from build123d import *

# Parameters (mm, degrees)
SKETCH1_R                = 150
BOSS_EXTRUDE1_DEPTH      = 75
CHAMFER1_SIZE            = 10
BOSS_EXTRUDE2_START      = -65
BOSS_EXTRUDE2_DEPTH      = 10
CHAMFER2_SIZE            = 7
BOSS_EXTRUDE3_DEPTH      = 9
BOSS_EXTRUDE4_DEPTH      = 3.5
CIRPATTERN1_COUNT        = 4
CIRPATTERN1_COPY_1_DEPTH = 9
CIRPATTERN1_COPY_2_DEPTH = 9
CIRPATTERN1_COPY_3_DEPTH = 9
CIRPATTERN1_COPY_4_DEPTH = 3.5
CIRPATTERN1_COPY_5_DEPTH = 3.5
CIRPATTERN1_COPY_6_DEPTH = 3.5
CUT_EXTRUDE1_START       = -60
CUT_EXTRUDE1_DEPTH       = 60
SKETCH6_R                = 110
BOSS_EXTRUDE5_DEPTH      = 9
BOSS_EXTRUDE5_TAPER      = 45
SKETCH7_R                = 15
BOSS_EXTRUDE6_DEPTH      = 20


with BuildPart() as part:
    # Sketch1 → Boss-Extrude1 (new body)
    with BuildSketch(Plane(origin=(0, 0, 0), x_dir=(1, 0, 0), z_dir=(0, 1, 0))):
        with Locations(Location((0, 0, 0), (0, 0, 270))):
            Circle(SKETCH1_R)
    extrude(amount=BOSS_EXTRUDE1_DEPTH)

    # Chamfer1
    chamfer1_edges = [part.edges().sort_by_distance(p)[0] for p in [
        (0, 75, -150),
    ]]
    chamfer(chamfer1_edges, length=CHAMFER1_SIZE)

    # Sketch2 → Boss-Extrude2 (add)
    with BuildSketch(Plane(origin=(0, 75, 0), x_dir=(1, 0, 0), z_dir=(0, 1, 0)).offset(BOSS_EXTRUDE2_START)):
        with BuildLine():
            Line((-145.236875483, 37.5), (-195.236875483, 37.5))
            Line((-195.236875483, 37.5), (-195.236875483, -37.5))
            Line((-195.236875483, -37.5), (-145.236875483, -37.5))
            ThreePointArc((-145.236875483, -37.5), (-150, 0), (-145.236875483, 37.5))
        make_face()
    boss_extrude2 = extrude(amount=BOSS_EXTRUDE2_DEPTH)

    # Chamfer2
    chamfer2_edges = [part.edges().sort_by_distance(p)[0] for p in [
        (-195.236875483, 15, -37.5),
        (-195.236875483, 15, 37.5),
    ]]
    chamfer(chamfer2_edges, length=CHAMFER2_SIZE)

    # Sketch3 → Boss-Extrude3 (add)
    with BuildSketch(Plane.XY.offset(37.5)):
        Polygon((-145.236875483, 20), (-145.236875483, 65), (-170.556875483, 65), (-188.236875483, 20), align=None)
    boss_extrude3 = extrude(amount=-BOSS_EXTRUDE3_DEPTH)

    # Sketch4 → Boss-Extrude4 (add)
    with BuildSketch(Plane(origin=(0, 20, 0), x_dir=(1, 0, 0), z_dir=(0, 1, 0))):
        Polygon((-183.04072306, -12), (-188.236875483, -9), (-193.433027905, -12), (-193.433027905, -18), (-188.236875483, -21), (-183.04072306, -18), align=None)
    boss_extrude4 = extrude(amount=BOSS_EXTRUDE4_DEPTH)

    # Mirror1: Boss-Extrude3, Boss-Extrude4 across plane
    add(boss_extrude3.mirror(Plane.XY))
    add(boss_extrude4.mirror(Plane.XY))

    # CirPattern1: Boss-Extrude2, Boss-Extrude3, Boss-Extrude4 ×4 about axis
    cirpattern1_axis = Axis((0, 0, 0), (0, 1, 0))
    add([boss_extrude2.rotate(cirpattern1_axis, i * 360 / CIRPATTERN1_COUNT) for i in range(1, CIRPATTERN1_COUNT)])
    add([boss_extrude3.rotate(cirpattern1_axis, i * 360 / CIRPATTERN1_COUNT) for i in range(1, CIRPATTERN1_COUNT)])
    add([boss_extrude4.rotate(cirpattern1_axis, i * 360 / CIRPATTERN1_COUNT) for i in range(1, CIRPATTERN1_COUNT)])

    # CirPattern1 copy 1 sketch → CirPattern1 copy 1 (add)
    with BuildSketch(Plane(origin=(-37.5, 0, 0), x_dir=(0, 0, -1), z_dir=(-1, 0, 0))):
        Polygon((-145.236875483, -20), (-145.236875483, -65), (-170.556875483, -65), (-188.236875483, -20), align=None)
    extrude(amount=-CIRPATTERN1_COPY_1_DEPTH)

    # CirPattern1 copy 2 sketch → CirPattern1 copy 2 (add)
    with BuildSketch(Plane(origin=(0, 0, 37.5), x_dir=(-1, 0, 0), z_dir=(0, 0, 1))):
        Polygon((-145.236875483, -20), (-145.236875483, -65), (-170.556875483, -65), (-188.236875483, -20), align=None)
    extrude(amount=-CIRPATTERN1_COPY_2_DEPTH)

    # CirPattern1 copy 3 sketch → CirPattern1 copy 3 (add)
    with BuildSketch(Plane(origin=(37.5, 0, 0), x_dir=(0, 0, 1), z_dir=(1, 0, 0))):
        Polygon((-145.236875483, -20), (-145.236875483, -65), (-170.556875483, -65), (-188.236875483, -20), align=None)
    extrude(amount=-CIRPATTERN1_COPY_3_DEPTH)

    # CirPattern1 copy 4 sketch → CirPattern1 copy 4 (add)
    with BuildSketch(Plane(origin=(0, 20, 0), x_dir=(0, 0, -1), z_dir=(0, 1, 0))):
        Polygon((-183.04072306, 12), (-188.236875483, 9), (-193.433027905, 12), (-193.433027905, 18), (-188.236875483, 21), (-183.04072306, 18), align=None)
    extrude(amount=CIRPATTERN1_COPY_4_DEPTH)

    # CirPattern1 copy 5 sketch → CirPattern1 copy 5 (add)
    with BuildSketch(Plane(origin=(0, 20, 0), x_dir=(-1, 0, 0), z_dir=(0, 1, 0))):
        Polygon((-183.04072306, 12), (-188.236875483, 9), (-193.433027905, 12), (-193.433027905, 18), (-188.236875483, 21), (-183.04072306, 18), align=None)
    extrude(amount=CIRPATTERN1_COPY_5_DEPTH)

    # CirPattern1 copy 6 sketch → CirPattern1 copy 6 (add)
    with BuildSketch(Plane.ZX.offset(20)):
        Polygon((-183.04072306, 12), (-188.236875483, 9), (-193.433027905, 12), (-193.433027905, 18), (-188.236875483, 21), (-183.04072306, 18), align=None)
    extrude(amount=CIRPATTERN1_COPY_6_DEPTH)

    # Sketch5 → Cut-Extrude1 (cut)
    with BuildSketch(Plane(origin=(0, 75, 0), x_dir=(1, 0, 0), z_dir=(0, 1, 0)).offset(CUT_EXTRUDE1_START)):
        with BuildLine():
            Line((-112.583302492, -65), (-129.903810568, -75))
            ThreePointArc((-129.903810568, -75), (-106.066017178, -106.066017178), (-75, -129.903810568))
            Line((-75, -129.903810568), (-65, -112.583302492))
            ThreePointArc((-65, -112.583302492), (-91.923881554, -91.923881554), (-112.583302492, -65))
        make_face()
    extrude(amount=CUT_EXTRUDE1_DEPTH, mode=Mode.SUBTRACT)

    # Sketch6 → Boss-Extrude5 (add)
    with BuildSketch(Plane(origin=(0, 75, 0), x_dir=(1, 0, 0), z_dir=(0, 1, 0))):
        Circle(SKETCH6_R)
    extrude(amount=BOSS_EXTRUDE5_DEPTH, taper=BOSS_EXTRUDE5_TAPER)

    # Sketch7 → Boss-Extrude6 (add)
    with BuildSketch(Plane(origin=(0, 84, 0), x_dir=(1, 0, 0), z_dir=(0, 1, 0))):
        with Locations(Location((0, 0, 0), (0, 0, 270))):
            Circle(SKETCH7_R)
    extrude(amount=BOSS_EXTRUDE6_DEPTH)


solid = part.part
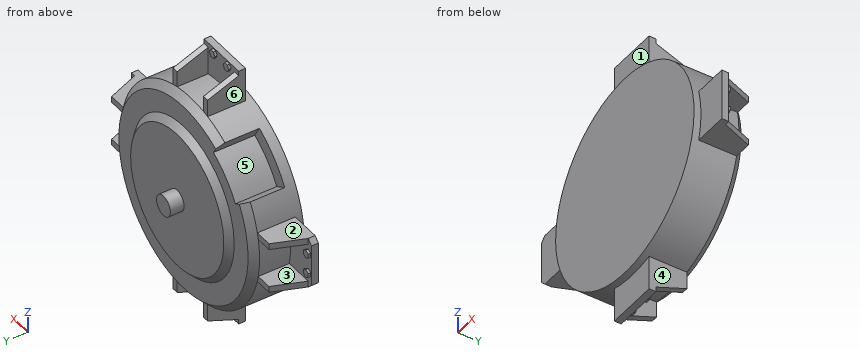
Geometry check sheet. Reference: the model listing, model coordinates, mm. Face numbers are marked on the shaded views. A direction names the side the tool comes from. Coordinates: 2 decimals unless noted, no trailing zeros. Order: outer loops, then holes, each group sorted by start corner. A loop starts at its lowest first (then second) coordinate and runs counter-clockwise, first axis right, second up. Notation, with made-up numbers: (62.25, 29) - (99.25, 29) arc R19 cw to (99.25, 35) - close; hole circle Ø10 at (0, 58.25). An arc over 180 degrees is marked (long way). One line per item, written item: value.
(1) Sectioned sample at B-B (y = 96.5). Enter the section's corners in (x, z), and give its area (3 significant figures).
Data:
outline: circle Ø30 at (0, 0)
area: 707 mm^2
(2) Access from +Z, -Z, +X, -X, +Y, -Y to the whole of each face (thin tool, end or side, straight path). Record for the marked faces 4, 5 and 6.
Data:
face 4: -Z, +X, +Y, -Y
face 5: +Y
face 6: +Z, -X, +Y, -Y
(3) Thickness scan on probe 1 along X at (y, z) = (22.5, 20); probe 2 along Z at (x, y) = (172.5, 39.5); probe 3 along Y at (x, z) = (34, -69). Record the ranges inside material, lowest first. Write a range as from..to.
Data:
probe 1: x = -189.97..-186.5, -148.66..148.66, 186.5..189.97
probe 2: z = -37.5..-28.5, 28.5..37.5
probe 3: y = 0..84
(4) Release check for a two-part mould opening along Z. For the marked faces 1, 2 and 3 record: +Z half, -Z half, draft (parallel to the pull), parting line (faces both ways), or undercut.
Data:
face 1: draft
face 2: +Z half
face 3: undercut
(5) Depth check by flat-ended pin: pin 1 Ø3 at (x, y) = (27.5, 46.5) entering from +Z; pin 2 Ø2.5 at (x, z) = (-160, 34) entering from +Y; pin 3 Ø12.5 at (x, y) = (-159.5, 43) entering from +Z. Enter the tip coordinate at first touch or a pass-through.
Data:
pin 1: stops at z = 178.26
pin 2: stops at y = 65
pin 3: stops at z = 37.5
(6) Sectioned sample at A-A (x = 0). Enter the section's corners in (y, z).
Data:
outline: (0, -150) - (10, -150) - (10, -195.24) - (20, -195.24) - (20, -150) - (65, -150) - (75, -140) - (75, -110) - (84, -101) - (84, -15) - (104, -15) - (104, 15) - (84, 15) - (84, 101) - (75, 110) - (75, 140) - (65, 150) - (20, 150) - (20, 195.24) - (10, 195.24) - (10, 150) - (0, 150) - close
